Verification items for the finished model (mm, model axes). Face numbers are marked on the shaded views. A direction names the side the tool comes from. Round coordinates to 2 decimals unless told otherwise and drop trailing zeros. Order: outer loops, then holes, each group sorted by start corner. A loop starts at its lowest first (then second) coordinate and runs counter-clockwise, first axis right, second up. Notation, with made-up numbers: (-25, -24) -> (21, -24) arc R18 ccw to (21, -8) -> close; hole circle Ø3 at (66.5, -15). An arc over 180 degrees is marked (long way). Put each result on its own line as item: value.
from build123d import *

# Parameters (mm, degrees)
F0_W     = 147.0372378826
F0_H     = 85.4446366429
F0_W_2   = 142.748
F0_H_2   = 2.1700232911
F0_H_3   = 4.2537826065
F0_H_4   = 2.8852941023
F1_DEPTH = 58.42
F0_H_5   = 23.8125
F0_H_6   = 23.8252
F2_DEPTH = 1.27
F3_W     = 1.6002
F3_H     = 17.4752
F4_DEPTH = 12.7
F5_W     = 3.175
F5_H     = 12.7
F6_DEPTH = 25.4


with BuildPart() as f1:
    # F0 (on Top) → F1 (new body)
    with BuildSketch(Plane.XY):
        Rectangle(F0_W, F0_H)
        Polygon((71.374, -37.5007058977), (71.374, -40.386), (-71.374, -40.386), (-71.374, -37.5007058977), (-71.374, -13.6755058977), (-71.374, -9.4217232911), (-71.374, 14.4034767089), (-71.374, 16.5735), (-71.374, 40.386), (71.374, 40.386), (71.374, 16.5735), (71.374, 14.4034767089), (71.374, -9.4217232911), (71.374, -13.6755058977), align=None, mode=Mode.SUBTRACT)
        with Locations((0, 15.4884883544)):
            Rectangle(F0_W_2, F0_H_2)
        with Locations((0, -11.5486145944)):
            Rectangle(F0_W_2, F0_H_3)
        with Locations((0, -38.9433529488)):
            Rectangle(F0_W_2, F0_H_4)
    extrude(amount=F1_DEPTH)

    # F0 (on Top) → F2 (join)
    with BuildSketch(Plane.XY):
        Rectangle(F0_W, F0_H)
        Polygon((71.374, -37.5007058977), (71.374, -40.386), (-71.374, -40.386), (-71.374, -37.5007058977), (-71.374, -13.6755058977), (-71.374, -9.4217232911), (-71.374, 14.4034767089), (-71.374, 16.5735), (-71.374, 40.386), (71.374, 40.386), (71.374, 16.5735), (71.374, 14.4034767089), (71.374, -9.4217232911), (71.374, -13.6755058977), align=None, mode=Mode.SUBTRACT)
        with Locations((0, 28.47975)):
            Rectangle(F0_W_2, F0_H_5)
        with Locations((0, 2.4908767089)):
            Rectangle(F0_W_2, F0_H_6)
        with Locations((0, -25.5881058977)):
            Rectangle(F0_W_2, F0_H_6)
    extrude(amount=F2_DEPTH)

    # F3 (on face) → F4 (join)
    with BuildSketch(Plane(origin=(-73.5186189413, 0, 0), x_dir=(0, -1, 0), z_dir=(-1, 0, 0))):
        with Locations((-9.0124478253, 49.6824)):
            Rectangle(F3_W, F3_H)
        with Locations((2.1127521747, 49.6824)):
            Rectangle(F3_W, F3_H)
    extrude(amount=F4_DEPTH)

    # F5 (on face) → F6 (cut)
    with BuildSketch(Plane(origin=(0, 9.8125478253, 0), x_dir=(-1, 0, 0), z_dir=(0, 1, 0))):
        with Locations((75.1061189413, 47.2948)):
            Rectangle(F5_W, F5_H)
    extrude(amount=-F6_DEPTH, mode=Mode.SUBTRACT)


solid = f1.part
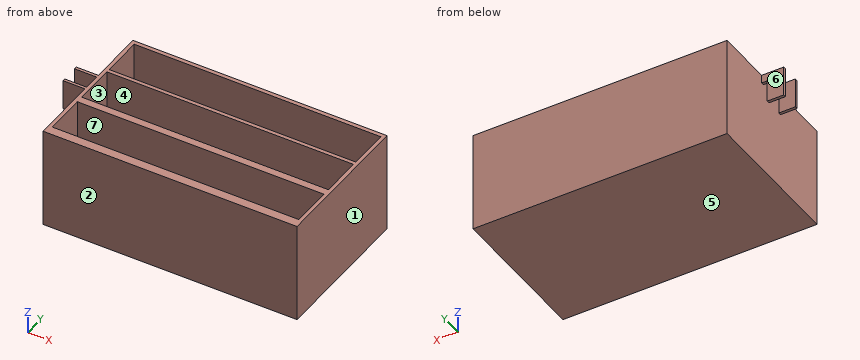
Item 1: Tool access check on the marked faces 5, 6 and 7. Record the directions out of +Z, -Z, +X, -X, +Y, -Y that give a thin tool (end or side, any length) a straight path to the whole face; none if there is none.
Check sheet entries:
face 5: -Z, +X, -X, +Y, -Y
face 6: +Z, -Z, -X, +Y
face 7: +Z
Item 2: Release check for a two-part mould opening along X. For the marked faces 1, 2, 3 and 4 record: +X half, -X half, draft (parallel to the pull), parting line (faces both ways), or undercut.
Check sheet entries:
face 1: +X half
face 2: draft
face 3: undercut
face 4: undercut
Item 3: Material ranges on L1, parallel to Y at x = 55, z = 12; L2, parallel to X at y = 28, z = 25; L3, parallel to Z at x = 52, y = -32, recorded low to high. Write a range as [from, to].
Check sheet entries:
L1: y = [-42.72, -37.5], [-13.68, -9.42], [14.4, 16.57], [40.39, 42.72]
L2: x = [-73.52, -71.37], [71.37, 73.52]
L3: z = [0, 1.27]
Item 4: Gauge pin test, flat ends, axial feed: pin 1 Ø10 at (x, y) = (-39.5, 11.5) entering from +Z; pin 2 Ø12 at (y, z) = (31, 38.5) entering from -X; pin 3 Ø6.5 at (x, z) = (-77, 46.5) entering from +Y; pin 4 Ø0.8 at (x, y) = (-82.5, -2) entering from -Z. Record the tip position at first contact, or that the pin passes through.
Check sheet entries:
pin 1: stops at z = 58.42
pin 2: stops at x = -73.52
pin 3: stops at y = 9.81
pin 4: stops at z = 40.94
Item 5: Section check C-C on y = 32. Record the boundary of the cut face in (x, z), then the cut area to 3 significant figures.
Check sheet entries:
outline: (-73.52, 0) -> (73.52, 0) -> (73.52, 58.42) -> (71.37, 58.42) -> (71.37, 1.27) -> (-71.37, 1.27) -> (-71.37, 58.42) -> (-73.52, 58.42) -> close
area: 432 mm^2
Item 6: Section check D-D on x = 39. Record the boundary of the cut face in (y, z), then the cut area to 3 significant figures.
Check sheet entries:
outline: (-42.72, 0) -> (42.72, 0) -> (42.72, 58.42) -> (40.39, 58.42) -> (40.39, 1.27) -> (16.57, 1.27) -> (16.57, 58.42) -> (14.4, 58.42) -> (14.4, 1.27) -> (-9.42, 1.27) -> (-9.42, 58.42) -> (-13.68, 58.42) -> (-13.68, 1.27) -> (-37.5, 1.27) -> (-37.5, 58.42) -> (-42.72, 58.42) -> close
area: 908 mm^2
Item 7: Section check A-A on z = 44. Record the boundary of the cut face in (x, y).
Check sheet entries:
outline: (-86.22, -2.91) -> (-76.69, -2.91) -> (-76.69, -1.31) -> (-86.22, -1.31) -> close; (-86.22, 8.21) -> (-76.69, 8.21) -> (-76.69, 9.81) -> (-86.22, 9.81) -> close; (-73.52, -42.72) -> (73.52, -42.72) -> (73.52, 42.72) -> (-73.52, 42.72) -> close; hole (-71.37, -37.5) -> (71.37, -37.5) -> (71.37, -13.68) -> (-71.37, -13.68) -> close; hole (-71.37, -9.42) -> (71.37, -9.42) -> (71.37, 14.4) -> (-71.37, 14.4) -> close; hole (-71.37, 16.57) -> (71.37, 16.57) -> (71.37, 40.39) -> (-71.37, 40.39) -> close
Item 8: Section check B-B on z = 15. Record the boundary of the cut face in (x, y), then the cut area to 3 significant figures.
Check sheet entries:
outline: (-73.52, -42.72) -> (73.52, -42.72) -> (73.52, 42.72) -> (-73.52, 42.72) -> close; hole (-71.37, -37.5) -> (71.37, -37.5) -> (71.37, -13.68) -> (-71.37, -13.68) -> close; hole (-71.37, -9.42) -> (71.37, -9.42) -> (71.37, 14.4) -> (-71.37, 14.4) -> close; hole (-71.37, 16.57) -> (71.37, 16.57) -> (71.37, 40.39) -> (-71.37, 40.39) -> close
area: 2,360 mm^2
